Design review of the part shown in the three views and the two pictorial views. Dimensions are in mm from the part's minimum x, y and z. A direction names the side the tool comes from. Round coordinates to 2 decimals unless told otherwise and drop trailing zeros. Loops run counter-clockwise (first coordinate to the right, second up) from the corner with the lowest first, then second, coordinate; pieces in that order, holes last. Notation, with made-up numbers: M 46,5 L 66,5 A17 cw 66,17 Z; hole C 19.5,-29 d8. An arc over 180 degrees is marked long. One line per question, with ' | ' between items. Start each with the question number.
1) For pin 1 Ø4 at (x, z) = (4.4, 12.65) entering from +Y; pin 2 Ø10 at (x, y) = (14, 14.5) entering from -Z; pin 3 Ø2.5 at (x, y) = (12.5, 59.5) entering from -Z; pin 4 Ø2 at (y, z) = (54.5, 17) entering from +X, all flat-tipped, find the tip position at first contact; note any pin that passes through.
2) We need section B-B (y = 34.5). Give the boundary of the cut face in (x, z).
3) For the marked faces 1, 2 and 3, list the 3-axis set-ups (+Z, -Z, +X, -X, +Y, -Y) from which the entire face can be reached by the end or side of a thin tool; tool diameter is ignored.
4) For probe 1 along X at (y, z) = (45.45, 12.65); probe 2 along Y at (x, z) = (17.75, 9.25); probe 3 along Y at (x, z) = (19.75, 2.5), list the stretches that pass through material, from the lowest coordinate up. Write a range as from..to.
5) We need section A-A (z = 12.65). Give the boundary of the cut face in (x, y), and give its area (3 significant figures).
6) We need section D-D (y = 49). Give the boundary of the cut face in (x, z), and give its area (3 significant figures).
7) We need section C-C (x = 12). Give the boundary of the cut face in (y, z).
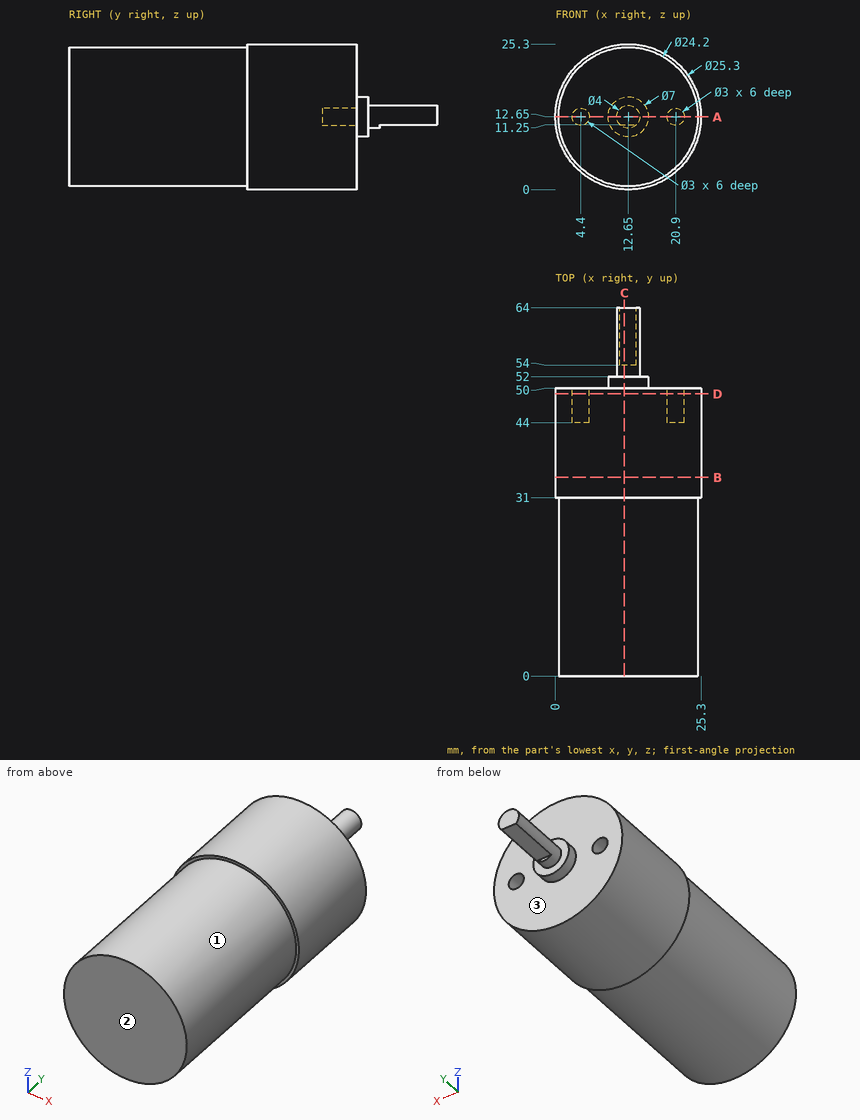
Answers below:
1) pin 1: y = 50 | pin 2: z = 0.55 | pin 3: z = 11.25 | pin 4: through
2) outline: C 12.65,12.65 d25.3
3) face 1: -Y | face 2: +Z, -Z, +X, -X, -Y | face 3: +Y
4) probe 1: 0..2.9, 5.9..19.4, 22.4..25.3 | probe 2: 0..50 | probe 3: 31..50
5) outline: M 0,31 L 0.55,31 L 0.55,0 L 24.75,0 L 24.75,31 L 25.3,31 L 25.3,50 L 22.4,50 L 22.4,44 L 19.4,44 L 19.4,50 L 16.15,50 L 16.15,52 L 14.65,52 L 14.65,64 L 10.65,64 L 10.65,52 L 9.15,52 L 9.15,50 L 5.9,50 L 5.9,44 L 2.9,44 L 2.9,50 L 0,50 Z | area: 1,260 mm^2
6) outline: C 12.65,12.65 d25.3; hole C 4.4,12.65 d3; hole C 20.9,12.65 d3 | area: 489 mm^2
7) outline: M 0,0.57 L 31,0.57 L 31,0.02 L 50,0.02 L 50,9.21 L 52,9.21 L 52,10.76 L 54,10.76 L 54,11.25 L 64,11.25 L 64,14.54 L 52,14.54 L 52,16.09 L 50,16.09 L 50,25.28 L 31,25.28 L 31,24.73 L 0,24.73 Z
